Verification items for the finished model (mm, model axes). Round coordinates to 2 decimals unless told otherwise and drop trailing zeros. Order: outer loops, then holes, each group sorted by start corner. A loop starts at its lowest first (then second) coordinate and runs counter-clockwise, first axis right, second up. Notation, with made-up numbers: M 33,76.25 L 58,76.25 A24 ccw 58,91.25 Z; hole C 11,-22.75 d5. An arc over 180 degrees is marked long. Return JSON: item names as keys, results as strings. Group by question number.
from build123d import *

# Parameters (mm, degrees)
SKETCH1_W           = 200
SKETCH1_H           = 80
BOSS_EXTRUDE1_DEPTH = 3
SKETCH2_R           = 2
CUT_EXTRUDE1_DEPTH  = 108.745069493
FILLET1_R           = 10
SKETCH3_R           = 1.560556943
CUT_EXTRUDE2_DEPTH  = 108.745069493
CUT_EXTRUDE3_DEPTH  = 108.745069493


with BuildPart() as part:
    # Sketch1 → Boss-Extrude1 (new body)
    with BuildSketch(Plane.XY):
        Rectangle(SKETCH1_W, SKETCH1_H)
    extrude(amount=BOSS_EXTRUDE1_DEPTH)

    # Sketch2 → Cut-Extrude1 (cut, through all)
    with BuildSketch(Plane.XY.offset(3)):
        with Locations((-92, 32)):
            Circle(SKETCH2_R)
        with Locations(Location((-92, -32, 0), (0, 0, 180))):
            Circle(SKETCH2_R)
        with Locations((92, -32)):
            Circle(SKETCH2_R)
        with Locations(Location((92, 32, 0), (0, 0, 180))):
            Circle(SKETCH2_R)
    extrude(amount=-CUT_EXTRUDE1_DEPTH, mode=Mode.SUBTRACT)

    # Fillet1
    fillet1_edges = [part.edges().sort_by_distance(p)[0] for p in [
        (100, -40, 1.5),
        (-100, -40, 1.5),
        (-100, 40, 1.5),
        (100, 40, 1.5),
    ]]
    fillet(fillet1_edges, radius=FILLET1_R)

    # Sketch3 → Cut-Extrude2 (cut, through all)
    with BuildSketch(Plane(origin=(0, 0, 0), x_dir=(-1, 0, 0), z_dir=(0, 0, -1))):
        with Locations((89.2, -8.5)):
            Circle(SKETCH3_R)
        with Locations((75.2, -8.5)):
            Circle(SKETCH3_R)
        with Locations((75.2, 8.5)):
            Circle(SKETCH3_R)
        with Locations((89.2, 8.5)):
            Circle(SKETCH3_R)
        with Locations((-89.2, -8.5)):
            Circle(SKETCH3_R)
        with Locations((-75.2, -8.5)):
            Circle(SKETCH3_R)
        with Locations((-89.2, 8.5)):
            Circle(SKETCH3_R)
        with Locations((-75.2, 8.5)):
            Circle(SKETCH3_R)
    extrude(amount=-CUT_EXTRUDE2_DEPTH, mode=Mode.SUBTRACT)

    # Sketch4 → Cut-Extrude3 (cut, through all)
    with BuildSketch(Plane.XY.offset(3)):
        with BuildLine():
            Line((15, 30), (-15, 30))
            ThreePointArc((-15, 30), (-18, 33), (-15, 36))
            Line((-15, 36), (15, 36))
            ThreePointArc((15, 36), (18, 33), (15, 30))
        make_face()
        with BuildLine():
            Line((15, -30), (-15, -30))
            ThreePointArc((-15, -30), (-18, -33), (-15, -36))
            Line((-15, -36), (15, -36))
            ThreePointArc((15, -36), (18, -33), (15, -30))
        make_face()
    extrude(amount=-CUT_EXTRUDE3_DEPTH, mode=Mode.SUBTRACT)


solid = part.part
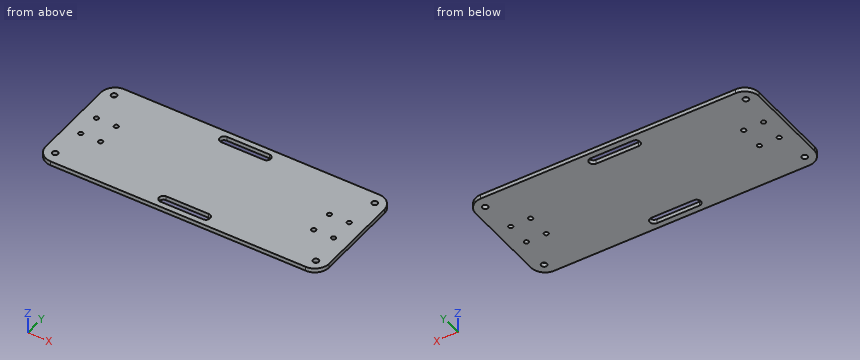
1. Thickness scan on line 1 along Y through (x, z) = (-2, 2.5); line 2 along Y through (x, z) = (89.2, 0.8). Record the ranges inside material, lowest first. Write a range as from..to.
2. Cross-section at A-A (z = 0.85). Give the number of separate pieces and of enclosed holes in the cut face, plus the area to 3 significant figures.
3. Cross-section at B-B (y = -32). Enter the section's corners in (x, z).
Computed:
{
 "1": {"line 1": "y = -40..-36, -30..30, 36..40", "line 2": "y = -40..-10.06, -6.94..6.94, 10.06..40"},
 "2": {"separate pieces": "1", "enclosed holes": "14", "area": "15,400 mm²"},
 "3": {"outline": "M -99.8,0 L -94,0 L -94,3 L -99.8,3 Z; M -90,0 L -17.83,0 L -17.83,3 L -90,3 Z; M 17.83,0 L 90,0 L 90,3 L 17.83,3 Z; M 94,0 L 99.8,0 L 99.8,3 L 94,3 Z"}
}
